from build123d import *

# Parameters (mm, degrees)
ESQUISSE1_R              = 2
BASE_RECTANGULAIRE_DEPTH = 38
ESQUISSE2_R              = 11
BOSS_DISQUE_DEPTH        = 2
ESQUISSE3_R              = 3
BOSS_AXE_DEPTH           = 22


with BuildPart() as part:
    # Esquisse1 → BASE RECTANGULAIRE (new body)
    with BuildSketch(Plane.XY):
        Polygon((-19.15, -21.15), (19.15, -21.15), (21.15, -19.15), (21.15, 19.15), (19.15, 21.15), (-19.15, 21.15), (-21.15, 19.15), (-21.15, -19.15), align=None)
        with Locations((-15.5, 15.5)):
            Circle(ESQUISSE1_R, mode=Mode.SUBTRACT)
        with Locations(Location((15.5, 15.5, 0), (0, 0, 180))):
            Circle(ESQUISSE1_R, mode=Mode.SUBTRACT)
        with Locations((15.5, -15.5)):
            Circle(ESQUISSE1_R, mode=Mode.SUBTRACT)
        with Locations(Location((-15.5, -15.5, 0), (0, 0, 180))):
            Circle(ESQUISSE1_R, mode=Mode.SUBTRACT)
    extrude(amount=BASE_RECTANGULAIRE_DEPTH)

    # Esquisse2 → BOSS DISQUE (add)
    with BuildSketch(Plane.XY.offset(38)):
        Circle(ESQUISSE2_R)
    extrude(amount=BOSS_DISQUE_DEPTH)

    # Esquisse3 → BOSS AXE (add)
    with BuildSketch(Plane.XY.offset(40)):
        Circle(ESQUISSE3_R)
    extrude(amount=BOSS_AXE_DEPTH)


solid = part.part
Here's how the part is built. I have some questions about the finished solid (model axes, mm). A direction names the side the tool comes from. Round coordinates to 2 decimals unless told otherwise and drop trailing zeros. Loops run counter-clockwise (first coordinate to the right, second up) from the corner with the lowest first, then second, coordinate; pieces in that order, holes last. Notation, with made-up numbers: (-12, 3) -> (40, 3) arc R22 ccw to (40, 34) -> close; hole circle Ø6 at (71, 56.5). An arc over 180 degrees is marked (long way). Write each question's results on one line, items separated by ' | '.
(1) If we section it at B-B, the plane y = -15.5: List the corners of the cut face in (x, z) for me.
Worked answers:
outline: (-21.15, 0) -> (-17.5, 0) -> (-17.5, 38) -> (-21.15, 38) -> close; (-13.5, 0) -> (13.5, 0) -> (13.5, 38) -> (-13.5, 38) -> close; (17.5, 0) -> (21.15, 0) -> (21.15, 38) -> (17.5, 38) -> close
(2) If we section it at D-D, the plane y = 0: List the corners of the cut face in (x, z) for me.
Worked answers:
outline: (-21.15, 0) -> (21.15, 0) -> (21.15, 38) -> (11, 38) -> (11, 40) -> (3, 40) -> (3, 62) -> (-3, 62) -> (-3, 40) -> (-11, 40) -> (-11, 38) -> (-21.15, 38) -> close
(3) For faces 5 (the face through (-3, 0, 51)), 6 (the face through (-15.76, 17.483, 18.734)), which set-ups out of +Z, -Z, +X, -X, +Y, -Y let a thin tool reach every point of the face, with its end or its side?
Worked answers:
face 5: +Z | face 6: +Z, -Z
(4) For P1, Ø3, axis at x = -15.5, y = 15.5, coming from the +Z side; P2, Ø3, axis at x = -0.5, y = 14, coming from the +Z side; P3, Ø12.5, axis at x = 3, y = 10.5, coming from the +Z side; P4, Ø3, axis at x = 7, z = 40, coming from the +Y side, each with a flat end and sliding along its axis, tell me the tip position at first contact or that it passes through.
Worked answers:
P1: through | P2: z = 38 | P3: z = 40 | P4: y = 9.53
(5) We'd pull the mould along Y, two halves only. Please class faces 1 (the face through (0, -21.15, 19)), 2 (the face through (-15.24, -17.483, 18.734)), 3 (the face through (20.2, 20.1, 18.7)), 4 (the face through (0, 0, 62)): released by +Y, released by -Y, zero draft, split by the parting line, or undercut.
Worked answers:
face 1: released by -Y | face 2: undercut | face 3: released by +Y | face 4: zero draft
(6) If we section it at A-A, the plane z = 21.5: List the corners of the cut face in (x, y) for me.
Worked answers:
outline: (-21.15, -19.15) -> (-19.15, -21.15) -> (19.15, -21.15) -> (21.15, -19.15) -> (21.15, 19.15) -> (19.15, 21.15) -> (-19.15, 21.15) -> (-21.15, 19.15) -> close; hole circle Ø4 at (-15.5, -15.5); hole circle Ø4 at (-15.5, 15.5); hole circle Ø4 at (15.5, -15.5); hole circle Ø4 at (15.5, 15.5)
(7) If I drill on L1, parallel to Y at x = 15.5, z = 9; L2, parallel to Y at x = 15, z = 29; L3, parallel to Z at x = 17, y = 9.5, over which ranges is the centre line in solid material (lowest first)?
Worked answers:
L1: -21.15 to -17.5, -13.5 to 13.5, 17.5 to 21.15 | L2: -21.15 to -17.44, -13.56 to 13.56, 17.44 to 21.15 | L3: 0 to 38
